Part model, mm, in its own coordinate system. A direction names the side the tool comes from. Give positions to 0.01 mm unless a question says otherwise; leave off trailing zeros. Order: outer loops, then holes, each group sorted by start corner. A loop starts at its lowest first (then second) coordinate and runs counter-clockwise, first axis right, second up.
from build123d import *

# Parameters (mm, degrees)
F0_W     = 45
F0_H     = 500
F1_DEPTH = 45
F2_W     = 15
F2_H     = 45
F3_DEPTH = 94
F4_W     = 15
F4_H     = 45
F5_DEPTH = 22.5


with BuildPart() as f1:
    # F0 (on Front) → F1 (new body)
    with BuildSketch(Plane.XZ):
        Rectangle(F0_W, F0_H)
    extrude(amount=F1_DEPTH)

    # F2 (on face) → F3 (cut)
    with BuildSketch(Plane.XZ.offset(45)):
        with Locations((0, 227.5)):
            Rectangle(F2_W, F2_H)
    extrude(amount=-F3_DEPTH, mode=Mode.SUBTRACT)

    # F4 (on Front) → F5 (cut)
    with BuildSketch(Plane.XZ):
        Rectangle(F4_W, F4_H)
    extrude(amount=F5_DEPTH, mode=Mode.SUBTRACT)


solid = f1.part
Item 1: Which spindle directions (+Z, -Z, +X, -X, +Y, -Y) get a long thin tool onto all of the face, cutting with end or side? Do faces 1 (the face through (-7.5, -23, 227)), 2 (the face through (-7.5, -11, 0)), 3 (the face through (0, -45, 4)). Say none if no direction does.
Item 2: Band-saw the part on A-A on x = 2. List the corners of the cut face in (y, z).
Item 3: Drill centre lines: probe 1 along X at (y, z) = (-19.5, -7); probe 2 along Z at (x, y) = (-1, -33). Where is each one in solid material? Low to high.
Item 4: Drop flat-ended pins along their axis: P1, Ø4.5, axis at x = 2, y = -6, coming from the +Z side; P2, Ø10, axis at x = 11.5, z = -71, coming from the +Y side; P3, Ø12, axis at x = -0.5, z = -3, coming from the +Y side. Give the stop position or say it passes through.
Item 5: Band-saw the part on B-B on y = -6.5. List the corners of the cut face in (x, z).
Item 6: Band-saw the part on C-C on z = -10. List the corners of the cut face in (x, y), plus the area to 3 significant figures.
Working result:
1. face 1: +Z, +Y, -Y
1. face 2: +Y
1. face 3: +Z, -Z, +X, -X, -Y
2. outline: (-45, -250) - (0, -250) - (0, -22.5) - (-22.5, -22.5) - (-22.5, 22.5) - (0, 22.5) - (0, 205) - (-45, 205) - close
3. probe 1: x = -22.5 to -7.5, 7.5 to 22.5
3. probe 2: z = -250 to 205
4. P1: stops at z = 205
4. P2: stops at y = 0
4. P3: stops at y = -22.5
5. outline: (-22.5, -250) - (22.5, -250) - (22.5, 250) - (7.5, 250) - (7.5, 205) - (-7.5, 205) - (-7.5, 250) - (-22.5, 250) - close; hole (-7.5, -22.5) - (7.5, -22.5) - (7.5, 22.5) - (-7.5, 22.5) - close
6. outline: (-22.5, -45) - (22.5, -45) - (22.5, 0) - (7.5, 0) - (7.5, -22.5) - (-7.5, -22.5) - (-7.5, 0) - (-22.5, 0) - close
6. area: 1,690 mm2
